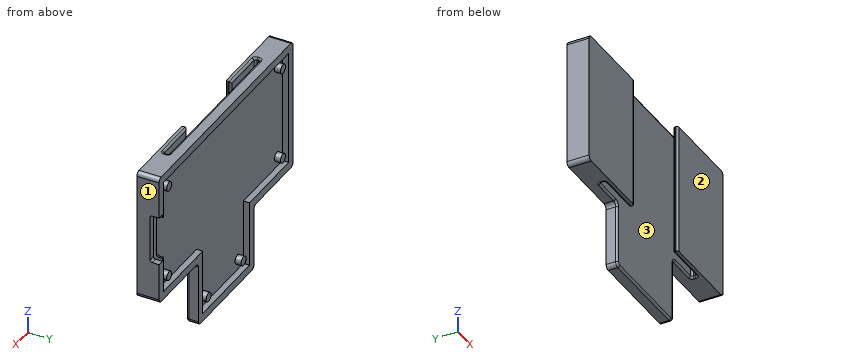
```python
from build123d import *

# Parameters (mm, degrees)
BOSS_EXTRUDE1_DEPTH     = 1.5
BOSS_EXTRUDE2_START     = 1.5
SKETCH2_3_R             = 1.125
BOSS_EXTRUDE2_DEPTH     = 1.5
BOSS_EXTRUDE3_DEPTH     = 2.5
FILLET1_R               = 1
CUT_EXTRUDE1_DEPTH      = 45.921292279
CUT_EXTRUDE1_DEPTH_BACK = 45.921292279
SKETCH3_W               = 42
SKETCH3_H               = 1.4
SKETCH3_W_2             = 20
SKETCH3_H_2             = 1.25
CUT_EXTRUDE3_START      = -16.35
SKETCH3_4_W             = 5
SKETCH3_4_H             = 1.25
SKETCH3_4_W_2           = 20
CUT_EXTRUDE3_DEPTH      = 29.571292279
FILLET2_R               = 0.5
CUT_EXTRUDE2_START      = 0.75
SKETCH2_5_W             = 1.5
SKETCH2_5_H             = 0.75
SKETCH2_5_H_2           = 10.7
CUT_EXTRUDE2_DEPTH      = 0.75
FILLET3_R               = 0.5


with BuildPart() as part:
    # Sketch2 → Boss-Extrude1 (new body)
    with BuildSketch(Plane(origin=(0, 0, 0), x_dir=(1, 0, 0), z_dir=(0, 1, 0))):
        Polygon((12.7, 16.35), (12.7, 32.75), (-12.7, 32.75), (-12.7, 16.35), (-30.6, 16.35), (-30.6, -16.35), (30.6, -16.35), (30.6, 16.35), align=None)
    extrude(amount=BOSS_EXTRUDE1_DEPTH)

    # Sketch2<3> → Boss-Extrude2 (add)
    with BuildSketch(Plane(origin=(0, 0, 0), x_dir=(1, 0, 0), z_dir=(0, 1, 0)).offset(BOSS_EXTRUDE2_START)):
        Polygon((-30.6, 16.35), (-30.6, -16.35), (30.6, -16.35), (30.6, -6.1), (29.1, -6.1), (29.1, -5.35), (28.6, -5.35), (28.6, -14.35), (-28.6, -14.35), (-28.6, 14.35), (-10.7, 14.35), (-10.7, 30.75), (10.7, 30.75), (10.7, 14.35), (28.6, 14.35), (28.6, 5.35), (29.1, 5.35), (29.1, 6.1), (30.6, 6.1), (30.6, 16.35), (12.7, 16.35), (12.7, 32.75), (-12.7, 32.75), (-12.7, 16.35), align=None)
        with Locations(Location((-26, 11.75, 0), (0, 0, 270))):
            Circle(SKETCH2_3_R)
        with Locations(Location((-26, -11.75, 0), (0, 0, 270))):
            Circle(SKETCH2_3_R)
        with Locations(Location((26, -11.75, 0), (0, 0, 270))):
            Circle(SKETCH2_3_R)
        with Locations(Location((26, 11.75, 0), (0, 0, 270))):
            Circle(SKETCH2_3_R)
        with Locations(Location((8, 28.05, 0), (0, 0, 270))):
            Circle(SKETCH2_3_R)
        with Locations(Location((-8, 28.05, 0), (0, 0, 270))):
            Circle(SKETCH2_3_R)
    extrude(amount=BOSS_EXTRUDE2_DEPTH)

    # Sketch2<4> → Boss-Extrude3 (add)
    with BuildSketch(Plane(origin=(0, 0, 0), x_dir=(1, 0, 0), z_dir=(0, 1, 0))):
        Polygon((12.7, 16.35), (12.7, 32.75), (-12.7, 32.75), (-12.7, 16.35), (-30.6, 16.35), (-30.6, -16.35), (30.6, -16.35), (30.6, 16.35), align=None)
    extrude(amount=-BOSS_EXTRUDE3_DEPTH)

    # Fillet1
    fillet1_edges = [part.edges().sort_by_distance(p)[0] for p in [
        (30.6, 0.25, 16.35),
        (-30.6, 0.25, 16.35),
        (-30.6, 0.25, -16.35),
        (-12.7, 0.25, -16.35),
        (-12.7, 0.25, -32.75),
        (12.7, 0.25, -32.75),
        (12.7, 0.25, -16.35),
        (30.6, 0.25, -16.35),
    ]]
    fillet(fillet1_edges, radius=FILLET1_R)

    # Sketch3 → Cut-Extrude1 (cut, two sides: drawn at the far end of the back side and taken through both)
    with BuildSketch(Plane.XY.offset(-CUT_EXTRUDE1_DEPTH_BACK)):
        with Locations((0, -0.55)):
            Rectangle(SKETCH3_W, SKETCH3_H)
        with Locations((0, -1.875)):
            Rectangle(SKETCH3_W_2, SKETCH3_H_2)
    extrude(amount=CUT_EXTRUDE1_DEPTH + CUT_EXTRUDE1_DEPTH_BACK, mode=Mode.SUBTRACT)

    # Sketch3<4> → Cut-Extrude3 (cut, through all)
    with BuildSketch(Plane.XY.offset(CUT_EXTRUDE3_START)):
        with Locations((12.5, -1.875)):
            Rectangle(SKETCH3_4_W, SKETCH3_4_H)
        with Locations((0, -1.875)):
            Rectangle(SKETCH3_4_W_2, SKETCH3_4_H)
        with Locations((-12.5, -1.875)):
            Rectangle(SKETCH3_4_W, SKETCH3_4_H)
    extrude(amount=-CUT_EXTRUDE3_DEPTH, mode=Mode.SUBTRACT)

    # Fillet2
    fillet2_edges = [part.edges().sort_by_distance(p)[0] for p in [
        (-12.407106781, 0.15, -32.457106781),
        (21, -0.55, -16.35),
        (15.5, -1.25, -16.35),
        (-15.5, -1.25, -16.35),
        (12.7, 0.15, -24.55),
        (12.992893219, 0.15, -16.642893219),
        (-12.992893219, 0.15, -16.642893219),
        (-21, -0.55, -16.35),
        (-21, -1.25, 0),
        (-21, -0.55, 16.35),
        (17.35, 0.15, -16.35),
        (12.407106781, 0.15, -32.457106781),
        (-12.7, 0.15, -24.55),
        (-17.35, 0.15, -16.35),
        (-21, 0.15, 0),
        (0, 0.15, 16.35),
        (21, 0.15, 0),
        (21, -1.25, 0),
        (0, 0.15, -32.75),
        (-15.5, -1.25, 16.35),
        (15.5, -1.25, 16.35),
        (21, -0.55, 16.35),
        (-10, -2.5, 0),
        (-10, -1.25, 0),
        (10, -1.25, 0),
        (10, -2.5, 0),
    ]]
    fillet(fillet2_edges, radius=FILLET2_R)

    # Sketch2<5> → Cut-Extrude2 (cut)
    with BuildSketch(Plane(origin=(0, 0, 0), x_dir=(1, 0, 0), z_dir=(0, 1, 0)).offset(CUT_EXTRUDE2_START)):
        with Locations((29.85, 5.725)):
            Rectangle(SKETCH2_5_W, SKETCH2_5_H)
        with Locations((29.85, 0)):
            Rectangle(SKETCH2_5_W, SKETCH2_5_H_2)
        with Locations((29.85, -5.725)):
            Rectangle(SKETCH2_5_W, SKETCH2_5_H)
    extrude(amount=CUT_EXTRUDE2_DEPTH, mode=Mode.SUBTRACT)

    # Fillet3
    fillet3_edges = [part.edges().sort_by_distance(p)[0] for p in [
        (29.85, 0.75, 6.1),
        (29.85, 0.75, -6.1),
        (28.85, 1.5, -5.35),
        (28.85, 1.5, 5.35),
    ]]
    fillet(fillet3_edges, radius=FILLET3_R)


solid = part.part
```
Design review of the part built by this model. Coordinates are the model's own, in mm. Face numbers are marked on the shaded views. Coordinates: 2 decimals unless noted, no trailing zeros. Loops run counter-clockwise (first coordinate to the right, second up) from the corner with the lowest first, then second, coordinate; pieces in that order, holes last. Notation, with made-up numbers: (-16, 32) -> (14, 32) arc R24 ccw to (14, 68) -> close; hole circle Ø10 at (38.25, 16.25). An arc over 180 degrees is marked (long way). Answer as a JSON object with one key per item and string values.
Q1. Take a section at B-B on z = -24. Give the boundary of the cut face in (x, y), plus the area to 3 significant figures.
Answer block:
{"outline": "(-12.7, 0.65) arc R0.5 ccw to (-12.2, 0.15) -> (12.2, 0.15) arc R0.5 ccw to (12.7, 0.65) -> (12.7, 3) -> (10.7, 3) -> (10.7, 1.5) -> (-10.7, 1.5) -> (-10.7, 3) -> (-12.7, 3) -> close", "area": "40.2 mm^2"}
Q2. The part is to be moulded in two halves that separate along Y. For the marked faces 1, 2 and 3, say which applies: +Y half, -Y half, draft (parallel to the pull), parting line (faces both ways), or undercut.
Answer block:
{"face 1": "draft", "face 2": "-Y half", "face 3": "undercut"}
Q3. Clearance check with flat-ended pins moving along their axes: pin 1 Ø2.5 at (y, z) = (2, -27) entering from +X; pin 2 Ø0.6 at (x, y) = (29, 2.5) entering from -Z; pin 3 Ø3 at (x, z) = (-18, -3) entering from +Y. State where each tip first meets the part, or that it passes through.
Answer block:
{"pin 1": "stops at x = 12.7", "pin 2": "stops at z = -16.35", "pin 3": "stops at y = 1.5"}
Q4. Take a section at C-C on x = 26. Give the boundary of the cut face in (y, z) (3 decimals), plus the area to 3 significant figures.
Answer block:
{"outline": "(-2.5, -16.35) -> (3, -16.35) -> (3, -14.35) -> (1.5, -14.35) -> (1.5, -12.875) -> (3, -12.875) -> (3, -10.625) -> (1.5, -10.625) -> (1.5, 10.625) -> (3, 10.625) -> (3, 12.875) -> (1.5, 12.875) -> (1.5, 14.35) -> (3, 14.35) -> (3, 16.35) -> (-2.5, 16.35) -> close", "area": "144 mm^2"}
Q5. To check wall thickness, follow L1, parallel to X at y = 1.65, z = 14; L2, parallel to Y at x = -17.5, z = -8.5; L3, parallel to Z at x = -14, y = 2.7. State the ranges of each line that lie inside material, in increasing order.
Answer block:
{"L1": "x = -30.6 to -28.6, 28.6 to 30.6", "L2": "y = -2.5 to -1.25, 0.15 to 1.5", "L3": "z = -16.35 to -14.35, 14.35 to 16.35"}
Q6. Take a section at A-A on x = 14.5. Give the boundary of the cut face in (y, z).
Answer block:
{"outline": "(-2.5, -16.35) -> (-1.75, -16.35) arc R0.5 ccw to (-1.25, -15.85) -> (-1.25, 15.85) arc R0.5 ccw to (-1.75, 16.35) -> (-2.5, 16.35) -> close; (0.15, -15.85) arc R0.5 ccw to (0.65, -16.35) -> (3, -16.35) -> (3, -14.35) -> (1.5, -14.35) -> (1.5, 14.35) -> (3, 14.35) -> (3, 16.35) -> (0.65, 16.35) arc R0.5 ccw to (0.15, 15.85) -> close"}
